from build123d import *

# Parameters (mm, degrees)
SKETCH1_W                               = 304.8
SKETCH1_H                               = 86.36
BOSS_EXTRUDE1_DEPTH                     = 3.175
F_1_8_0_125_PRESS_DOWEL_HOLE1_OUTLINE_R = 1.5875
F_1_8_0_125_PRESS_DOWEL_HOLE1_DEPTH     = 3.175
CUT_EXTRUDE1_DEPTH                      = 317.814094107
SKETCH7_W                               = 19.05
SKETCH7_H                               = 25.4
SKETCH7_H_2                             = 71.12
CUT_EXTRUDE2_DEPTH                      = 317.814094107
FILLET1_R                               = 3.175
F_1_2_0_5_PRESS_DOWEL_HOLE1_D           = 12.7
F_3_0MM_PRESS_DOWEL_HOLE1_D             = 3
F_3_0MM_PRESS_DOWEL_HOLE1_DEPTH         = 3.175
F_3_0MM_PRESS_DOWEL_HOLE1_TIP           = 0.901290929
F_2_0MM_PRESS_DOWEL_HOLE1_D             = 2
F_2_0MM_PRESS_DOWEL_HOLE1_DEPTH         = 3.175
F_2_0MM_PRESS_DOWEL_HOLE1_TIP           = 0.600860619
F_4_40_TAPPED_HOLE2_D                   = 2.2606
F_1_8_0_125_DIAMETER_HOLE1_D            = 3.175
F_4_CLEARANCE_HOLE1_D                   = 2.9464
F_4_CLEARANCE_HOLE1_DEPTH               = 9.1694
F_4_CLEARANCE_HOLE1_TIP                 = 0.885187864


# Read off the part's stored shape, not the designer's step: 1/8 (0.125) Press Dowel Hole1
with BuildPart() as part:
    # Sketch1 → Boss-Extrude1 (new body)
    with BuildSketch(Plane(origin=(0, 0, 0), x_dir=(0, 0, -1), z_dir=(1, 0, 0))):
        with Locations((152.4, 43.18)):
            Rectangle(SKETCH1_W, SKETCH1_H)
    extrude(amount=BOSS_EXTRUDE1_DEPTH)

    # 1/8 (0.125) Press Dowel Hole1 outline → 1/8 (0.125) Press Dowel Hole1 (cut)
    with BuildSketch(Plane.YZ):
        with Locations((68.36, -269.24)):
            Circle(F_1_8_0_125_PRESS_DOWEL_HOLE1_OUTLINE_R)
        with Locations((18, -269.24)):
            Circle(F_1_8_0_125_PRESS_DOWEL_HOLE1_OUTLINE_R)
        with Locations((82.55, -25.4)):
            Circle(F_1_8_0_125_PRESS_DOWEL_HOLE1_OUTLINE_R)
        with Locations((82.55, -88.9)):
            Circle(F_1_8_0_125_PRESS_DOWEL_HOLE1_OUTLINE_R)
        with Locations((82.55, -190.5)):
            Circle(F_1_8_0_125_PRESS_DOWEL_HOLE1_OUTLINE_R)
        with Locations((82.55, -254)):
            Circle(F_1_8_0_125_PRESS_DOWEL_HOLE1_OUTLINE_R)
        with Locations((3.81, -254)):
            Circle(F_1_8_0_125_PRESS_DOWEL_HOLE1_OUTLINE_R)
        with Locations((3.81, -190.5)):
            Circle(F_1_8_0_125_PRESS_DOWEL_HOLE1_OUTLINE_R)
        with Locations((3.81, -88.9)):
            Circle(F_1_8_0_125_PRESS_DOWEL_HOLE1_OUTLINE_R)
        with Locations((3.81, -25.4)):
            Circle(F_1_8_0_125_PRESS_DOWEL_HOLE1_OUTLINE_R)
    extrude(amount=F_1_8_0_125_PRESS_DOWEL_HOLE1_DEPTH, mode=Mode.SUBTRACT)

    # Sketch6 → Cut-Extrude1 (cut, through all)
    with BuildSketch(Plane(origin=(3.175, 0, 0), x_dir=(0, 0, -1), z_dir=(1, 0, 0))):
        with BuildLine():
            Line((141.5288, 73.66), (141.5288, 56.781492032))
            ThreePointArc((141.5288, 56.781492032), (139.7, 54.952692032), (137.8712, 56.781492032))
            Line((137.8712, 56.781492032), (137.8712, 73.66))
            ThreePointArc((137.8712, 73.66), (139.7, 75.4888), (141.5288, 73.66))
        make_face()
        with BuildLine():
            Line((141.5288, 12.7), (141.5288, 29.578507968))
            ThreePointArc((141.5288, 29.578507968), (139.7, 31.407307968), (137.8712, 29.578507968))
            Line((137.8712, 29.578507968), (137.8712, 12.7))
            ThreePointArc((137.8712, 12.7), (139.7, 10.8712), (141.5288, 12.7))
        make_face()
    extrude(amount=-CUT_EXTRUDE1_DEPTH, mode=Mode.SUBTRACT)

    # Sketch7 → Cut-Extrude2 (cut, through all)
    with BuildSketch(Plane(origin=(3.175, 0, 0), x_dir=(0, 0, -1), z_dir=(1, 0, 0))):
        Polygon((7.62, 73.66), (7.62, 12.7), (50.8, 43.18), align=None)
        with Locations((286.385, 66.04)):
            Rectangle(SKETCH7_W, SKETCH7_H)
        Polygon((100.33, 12.7), (57.15, 43.18), (100.33, 73.66), align=None)
        with Locations((161.925, 43.18)):
            Rectangle(SKETCH7_W, SKETCH7_H_2)
        Polygon((179.07, 25.4), (224.15112849, 43.18), (179.07, 60.96), align=None)
        Polygon((53.975, 73.66), (88.265, 73.66), (53.975, 49.455294118), (19.685, 73.66), align=None)
        Polygon((53.975, 36.904705882), (19.685, 12.7), (53.975, 12.7), (88.265, 12.7), align=None)
        Polygon((179.07, 12.7), (217.710967277, 27.94), (237.51919806, 27.94), (266.065, 19.05), (266.065, 12.7), (225.425, 12.7), align=None)
        Polygon((217.710967277, 58.42), (237.51919806, 58.42), (266.065, 67.31), (266.065, 73.66), (225.425, 73.66), (179.07, 73.66), align=None)
        with Locations((286.385, 20.32)):
            Rectangle(SKETCH7_W, SKETCH7_H)
        with Locations((117.475, 43.18)):
            Rectangle(SKETCH7_W, SKETCH7_H_2)
    extrude(amount=-CUT_EXTRUDE2_DEPTH, mode=Mode.SUBTRACT)

    # Fillet1
    fillet1_edges = [part.edges().sort_by_distance(p)[0] for p in [
        (1.5875, 73.66, -7.62),
        (1.5875, 43.18, -50.8),
        (1.5875, 12.7, -7.62),
        (1.5875, 53.34, -276.86),
        (1.5875, 78.74, -276.86),
        (1.5875, 78.74, -295.91),
        (1.5875, 53.34, -295.91),
        (1.5875, 73.66, -100.33),
        (1.5875, 12.7, -100.33),
        (1.5875, 43.18, -57.15),
        (1.5875, 12.7, -179.07),
        (1.5875, 27.94, -217.710967277),
        (1.5875, 27.94, -237.51919806),
        (1.5875, 19.05, -266.065),
        (1.5875, 12.7, -266.065),
        (1.5875, 25.4, -179.07),
        (1.5875, 60.96, -179.07),
        (1.5875, 43.18, -224.15112849),
        (1.5875, 73.66, -19.685),
        (1.5875, 73.66, -88.265),
        (1.5875, 49.455294118, -53.975),
        (1.5875, 36.904705882, -53.975),
        (1.5875, 12.7, -88.265),
        (1.5875, 12.7, -19.685),
        (1.5875, 73.66, -266.065),
        (1.5875, 67.31, -266.065),
        (1.5875, 58.42, -237.51919806),
        (1.5875, 58.42, -217.710967277),
        (1.5875, 73.66, -179.07),
        (1.5875, 7.62, -152.4),
        (1.5875, 78.74, -152.4),
        (1.5875, 78.74, -171.45),
        (1.5875, 7.62, -171.45),
        (1.5875, 7.62, -276.86),
        (1.5875, 33.02, -276.86),
        (1.5875, 33.02, -295.91),
        (1.5875, 7.62, -295.91),
        (1.5875, 7.62, -107.95),
        (1.5875, 78.74, -107.95),
        (1.5875, 78.74, -127),
        (1.5875, 7.62, -127),
    ]]
    fillet(fillet1_edges, radius=FILLET1_R)

    # 1/2 (0.5) Press Dowel Hole1 (through all)
    with Locations(Plane.ZY):
        with Locations((-248.01972494, 46.53348834)):
            Hole(F_1_2_0_5_PRESS_DOWEL_HOLE1_D / 2)

    # Ø3.0mm Press Dowel Hole1
    with Locations(Plane.ZY):
        with Locations((-253.55249518, 29.46260554)):
            Hole(F_3_0MM_PRESS_DOWEL_HOLE1_D / 2, depth=F_3_0MM_PRESS_DOWEL_HOLE1_DEPTH)
            with Locations((0, 0, -(F_3_0MM_PRESS_DOWEL_HOLE1_DEPTH + F_3_0MM_PRESS_DOWEL_HOLE1_TIP / 2))):  # 118° drill point
                Cone(0, F_3_0MM_PRESS_DOWEL_HOLE1_D / 2, F_3_0MM_PRESS_DOWEL_HOLE1_TIP, mode=Mode.SUBTRACT)

    # Ø2.0mm Press Dowel Hole1
    with Locations(Plane.ZY):
        with Locations((-267.20941224, 24.95127344)):
            Hole(F_2_0MM_PRESS_DOWEL_HOLE1_D / 2, depth=F_2_0MM_PRESS_DOWEL_HOLE1_DEPTH)
            with Locations((0, 0, -(F_2_0MM_PRESS_DOWEL_HOLE1_DEPTH + F_2_0MM_PRESS_DOWEL_HOLE1_TIP / 2))):  # 118° drill point
                Cone(0, F_2_0MM_PRESS_DOWEL_HOLE1_D / 2, F_2_0MM_PRESS_DOWEL_HOLE1_TIP, mode=Mode.SUBTRACT)

    # #4-40 Tapped Hole2 (through all)
    with Locations(Plane(origin=(3.175, 0, 0), x_dir=(0, 0, -1), z_dir=(1, 0, 0))):
        with Locations((301.625, 81.2038), (301.625, 5.1562), (3.175, 81.2038), (3.175, 5.1562), (175.26, 66.04), (175.26, 20.32), (104.14, 66.04), (104.14, 20.32), (5.1562, 12.7), (5.1562, 73.66), (299.6438, 73.66), (299.6438, 12.7)):
            Hole(F_4_40_TAPPED_HOLE2_D / 2)

    # 1/8 (0.125) Diameter Hole1 (through all)
    with Locations(Plane(origin=(3.175, 0, 0), x_dir=(0, 0, -1), z_dir=(1, 0, 0))):
        with Locations((278.835955069, 43.18)):
            Hole(F_1_8_0_125_DIAMETER_HOLE1_D / 2)

    # #4 Clearance Hole1
    with Locations(Plane(origin=(3.175, 0, 0), x_dir=(0, 0, -1), z_dir=(1, 0, 0))):
        with Locations((228.6, 81.2038), (63.5, 81.2038), (63.5, 5.1562), (241.3, 5.1562)):
            Hole(F_4_CLEARANCE_HOLE1_D / 2, depth=F_4_CLEARANCE_HOLE1_DEPTH)
            with Locations((0, 0, -(F_4_CLEARANCE_HOLE1_DEPTH + F_4_CLEARANCE_HOLE1_TIP / 2))):  # 118° drill point
                Cone(0, F_4_CLEARANCE_HOLE1_D / 2, F_4_CLEARANCE_HOLE1_TIP, mode=Mode.SUBTRACT)


solid = part.part
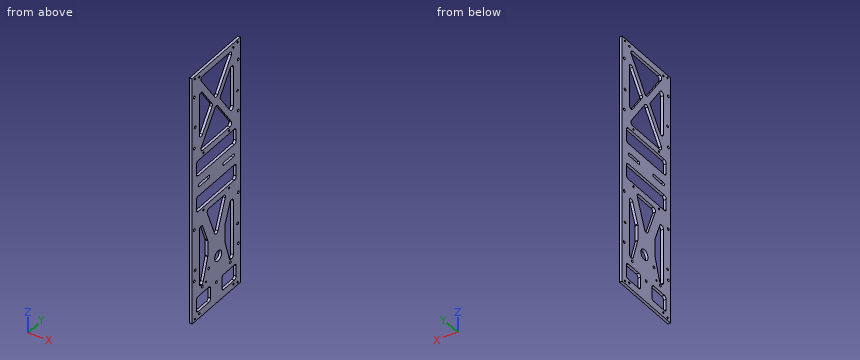
For this review, take the finished solid that the model builds, in its own axes (mm). Coordinates: 2 decimals unless noted, no trailing zeros. Write each loop counter-clockwise with the first axis right and the second up, starting at its lowest first coordinate (ties: lowest second). Pieces come first, ordered by that corner, then holes. Notation, with made-up numbers: (17, -18.5) -> (62, -18.5) arc R3 ccw to (62, -13.5) -> close; hole circle Ø7 at (74.25, 36). An arc over 180 degrees is marked (long way). Write each question's results on one line, items separated by ' | '. Start each with the question number.
1) Wall thickness on L1, parallel to Y at x = 2.1, z = -104.14; L2, parallel to Y at x = 1.4, z = -283; L3, parallel to Z at x = 1.4, y = 8: over which ranges is each line inside the solid? List them lowest first. Write a range as [from, to].
2) Consider section A-A (z = -35.5). Write out the cut boundary in (x, y) (3 decimals), plus the area to 3 significant figures.
3) Consider section B-B (x = 0.55). Give the number of separate pieces and of enclosed holes in the cut face, plus the area to 3 significant figures.
Geometry says:
1) L1: [0, 19.19], [21.45, 64.91], [67.17, 86.36] | L2: [0, 7.62], [33.02, 53.34], [78.74, 86.36] | L3: [-304.8, -294.24], [-278.53, -169.78], [-154.07, -125.33], [-109.62, 0]
2) outline: (0, 0) -> (3.175, 0) -> (3.175, 12.7) -> (0, 12.7) -> close; (0, 23.864) -> (3.175, 23.864) -> (3.175, 32.38) -> (0, 32.38) -> close; (0, 53.98) -> (3.175, 53.98) -> (3.175, 62.496) -> (0, 62.496) -> close; (0, 73.66) -> (3.175, 73.66) -> (3.175, 86.36) -> (0, 86.36) -> close | area: 135 mm^2
3) separate pieces: 1 | enclosed holes: 43 | area: 15,600 mm^2
